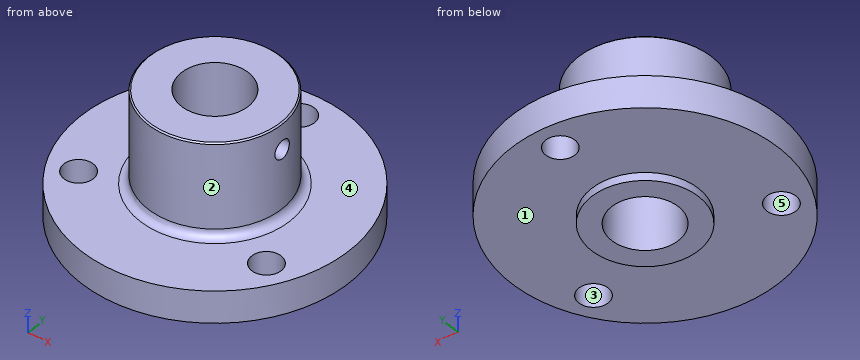
```python
from build123d import *

# Parameters (mm, degrees)
F2_R            = 3
F4_D            = 6.8
F4_DEPTH        = 50.001
F5_R            = 5.5
F6_DEPTH        = 15.0010001
F6_COPIES_COUNT = 3
F7_SIZE         = 0.5


# Not quite as in the source:
# - a pattern or mirror of a feature is missing from the dataset's text; its kind, count and spacing are read off the source's solid


with BuildPart() as f1:
    # F0 (on Front) → F1 (revolve)
    with BuildSketch(Plane.XZ):
        Polygon((-20, 0), (-12.5, 0), (-12.5, 50), (-25, 50), (-25, 15), (-50, 15), (-50, 3), (-20, 3), align=None)
    revolve(axis=Axis((0, 0, 33.7237479181), (0, 0, 1)))

    # F2
    f2_edges = [f1.edges().sort_by_distance(p)[0] for p in [
        (25, 0, 15),
    ]]
    fillet(f2_edges, radius=F2_R)

    # F4 (through all, one way)
    with BuildSketch(Plane(origin=(0, 0, 0), x_dir=(0, 1, 0), z_dir=(-1, 0, 0))):
        with Locations((0, -40)):
            Circle(F4_D / 2)
    extrude(amount=-F4_DEPTH, mode=Mode.SUBTRACT)

    # F5 (on face) → F6 (cut, through all)
    with BuildSketch(Plane.XY.offset(15)):
        with Locations((0, 40)):
            Circle(F5_R)
    f6 = extrude(amount=-F6_DEPTH, mode=Mode.SUBTRACT)

    # F6_copies: F6 ×3 about axis
    f6_copies_axis = Axis((0, 0, 0), (0, 0, 1))
    for i in range(1, F6_COPIES_COUNT):
        add(f6.rotate(f6_copies_axis, i * 360 / F6_COPIES_COUNT), mode=Mode.SUBTRACT)

    # F7
    f7_edges = [f1.edges().sort_by_distance(p)[0] for p in [
        (25, 0, 50),
    ]]
    chamfer(f7_edges, length=F7_SIZE)


solid = f1.part
```
Source: CAD feature listing. Evaluate the final solid. Frame: model axes, mm. Face numbers are marked on the shaded views. A direction names the side the tool comes from. Coordinates: 2 decimals unless noted, no trailing zeros. Loops run counter-clockwise (first coordinate to the right, second up) from the corner with the lowest first, then second, coordinate; pieces in that order, holes last. Notation, with made-up numbers: M -11,-11.5 L -2,-11.5 A21 ccw -2,13.5 Z; hole C -8.5,-17.75 d6. An arc over 180 degrees is marked long. Put each result on its own line as item: value. Start each with the question number.
1) Ray query, L1, parallel to Y at x = 0, z = 12; L2, parallel to X at y = 0, z = 20.5; L3, parallel to Z at x = 22.5, y = 0. Return the intervals inside material, ascending. Write a range as from..to.
2) Cut plane B-B on y = 40. Return the cut outline in (x, z).
3) Reachability of the marked faces 4 and 5 from +Z, -Z, +X, -X, +Y, -Y: full face, straight path, thin tool, end or side. Return the list, or none.
4) Cut plane A-A on x = 0. Return the cut outline in (y, z), then the cut area to 3 significant figures.
5) Cut plane D-D on z = 35. Return the cut outline in (x, y).
6) Cut plane C-C on y = 0. Return the cut outline in (x, z), then the cut area to 3 significant figures.
7) Pull-direction query (X, two-part tool) for the marked faces 1, 2 and 3; classes: pulls with the +X half, pulls with the -X half, needs draft (parallel to the pull), parting line crosses it, or undercut.
8) Contact query for flat-ended pins moving along their axis: pin 1 Ø12.5 at (x, y) = (-34.64, -20) entering from -Z; pin 2 Ø6 at (x, z) = (-15.5, 20.5) entering from -Y; pin 3 Ø8 at (y, z) = (-14, 38.5) entering from -X; pin 4 Ø1.5 at (x, y) = (3, 20.5) entering from -Z. Output: stop coordinate, or through.
The answers:
1. L1: y = -50..-12.5, 12.5..34.5, 45.5..50
1. L2: x = -25..-12.5, 12.5..25
1. L3: z = 3..36.6, 43.4..50
2. outline: M -30,3 L -5.5,3 L -5.5,15 L -30,15 Z; M 5.5,3 L 30,3 L 30,15 L 5.5,15 Z
3. face 4: +Z
3. face 5: +Z, -Z
4. outline: M -50,3 L -20,3 L -20,0 L -12.5,0 L -12.5,50 L -24.5,50 L -25,49.5 L -25,18 A3 cw -28,15 L -50,15 Z; M 12.5,0 L 20,0 L 20,3 L 34.5,3 L 34.5,15 L 28,15 A3 cw 25,18 L 25,49.5 L 24.5,50 L 12.5,50 Z; M 45.5,3 L 50,3 L 50,15 L 45.5,15 Z
4. area: 1,690 mm²
5. outline: C 0,0 d50; hole C 0,0 d25
6. outline: M -50,3 L -20,3 L -20,0 L -12.5,0 L -12.5,50 L -24.5,50 L -25,49.5 L -25,18 A3 cw -28,15 L -50,15 Z; M 12.5,0 L 20,0 L 20,3 L 50,3 L 50,15 L 28,15 A3 cw 25,18 L 25,36.6 L 12.5,36.6 Z; M 12.5,43.4 L 25,43.4 L 25,49.5 L 24.5,50 L 12.5,50 Z
6. area: 1,740 mm²
7. face 1: needs draft
7. face 2: parting line crosses it
7. face 3: undercut
8. pin 1: stops at z = 3
8. pin 2: stops at y = -21.65
8. pin 3: stops at x = -22.91
8. pin 4: stops at z = 0
